Source: three-view drawing plus pictorial views. Frame: mm from the lowest corner of the part. Give positions to 0.01 mm unless a question says otherwise; leave off trailing zeros. Order: outer loops, then holes, each group sorted by start corner. A loop starts at its lowest first (then second) coordinate and runs counter-clockwise, first axis right, second up. Notation, with made-up numbers: M 8.25,51 L 16.25,51 A30 ccw 16.25,74 Z; hole C 61,6.5 d9. An arc over 180 degrees is marked long. One line per question, with ' | ' between items. Start each with the question number.
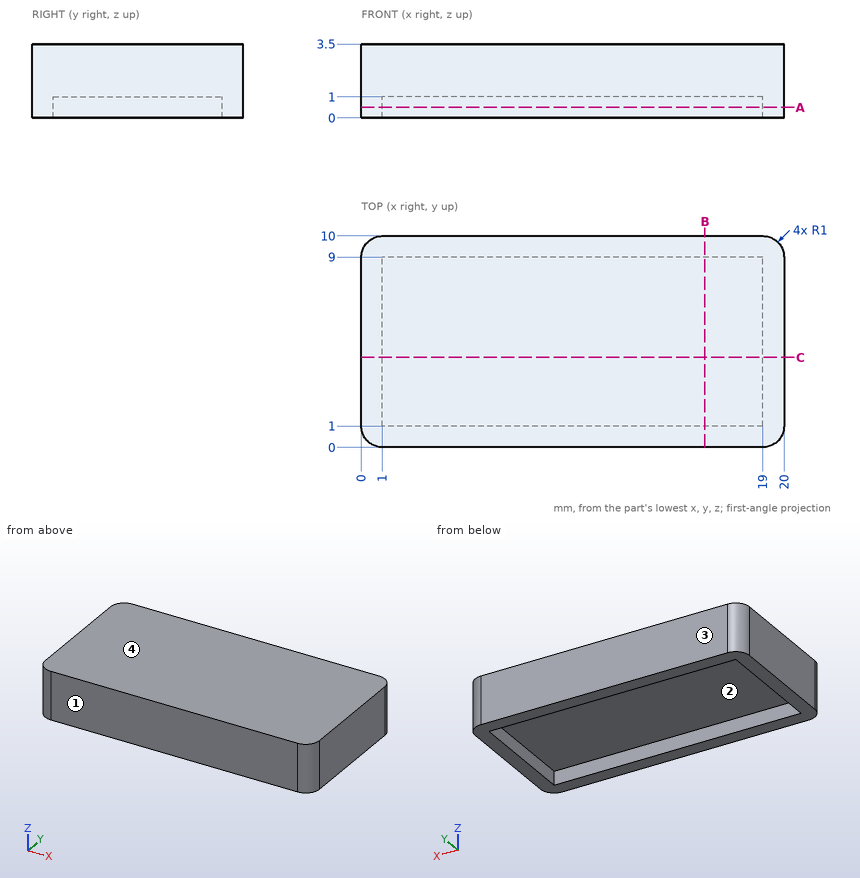
Item 1: Mould query, pull axis Y, two halves, no side actions, for the marked faces 1, 2, 3 and 4. Classes: pulls with the +Y half, pulls with the -Y half, needs draft (parallel to the pull), parting line crosses it, or undercut.
Item 2: Cut plane A-A on z = 0.5. Return the cut outline in (x, y), and give its area (3 significant figures).
Item 3: Line query: line 1 (Y direction, x = 15.5, z = 0.6); line 2 (X direction, y = 4.75, z = 0.8); line 3 (Z direction, x = 12.25, y = 7.25). Output: solid intervals per line, ascending.
Item 4: Cut plane B-B on x = 16.25. Return the cut outline in (y, z).
Item 5: Cut plane C-C on y = 4.25. Return the cut outline in (x, z), and give its area (3 significant figures).
Item 6: Pin query (flat end, axial travel): pin 1 Ø2 at (x, y) = (9.5, 4.5) entering from -Z; pin 2 Ø1.1 at (y, z) = (4.5, 0.5) entering from -X. Return the tip coordinate at first contact, or that it passes through.
Results are:
1) face 1: pulls with the -Y half | face 2: undercut | face 3: pulls with the +Y half | face 4: needs draft
2) outline: M 0,1 A1 ccw 1,0 L 19,0 A1 ccw 20,1 L 20,9 A1 ccw 19,10 L 1,10 A1 ccw 0,9 Z; hole M 1,1 L 19,1 L 19,9 L 1,9 Z | area: 55.1 mm2
3) line 1: y = 0 to 1, 9 to 10 | line 2: x = 0 to 1, 19 to 20 | line 3: z = 1 to 3.5
4) outline: M 0,0 L 1,0 L 1,1 L 9,1 L 9,0 L 10,0 L 10,3.5 L 0,3.5 Z
5) outline: M 0,0 L 1,0 L 1,1 L 19,1 L 19,0 L 20,0 L 20,3.5 L 0,3.5 Z | area: 52.0 mm2
6) pin 1: stops at z = 1 | pin 2: stops at x = 0
